Part model, mm, in its own coordinate system. Face numbers are marked on the shaded views. A direction names the side the tool comes from. Round coordinates to 2 decimals unless told otherwise and drop trailing zeros. Loops run counter-clockwise (first coordinate to the right, second up) from the corner with the lowest first, then second, coordinate; pieces in that order, holes last.
(1) Tool access for the marked faces 4, 5 and 6: list every direction of +Z, -Z, +X, -X, +Y, -Y with a clear straight run to the whole face (end or side of a thin tool).
(2) Cut at C-C on x = 13. List the corners of the cut face in (y, z) (3 decimals), then the cut area to 3 significant figures.
(3) Mould opens along X. For the marked faces 1, 2 and 3 say: +X half, -X half, draft (parallel to the pull), parting line (faces both ways), or undercut.
(4) Cut at A-A on z = 7. List the corners of the cut face in (x, y) (3 decimals).
(5) Flat gauge pins, fed straight in: pin 1 (4 mm diameter, centred on x = 10, z = -18, fed in from +Y); pin 2 (0.5 mm diameter, centred on x = -16.5, z = 37, fed in from +Y); pin 3 (1.7 mm diameter, centred on x = -21, z = -35, fed in from +Y). Where does each tip first touch, or does it go through?
(6) Cut at B-B on y = -8. Count the separate pieces of the cut face and the enclosed holes in it, then the cut area to 3 significant figures.
(7) Probe probe 1 along X at (y, z) = (-3.75, 4); probe 2 along Z at (x, y) = (0, -5.5); probe 3 along Z at (x, y) = (-20, -6.25). List the from-to ranges inside material, lowest first.
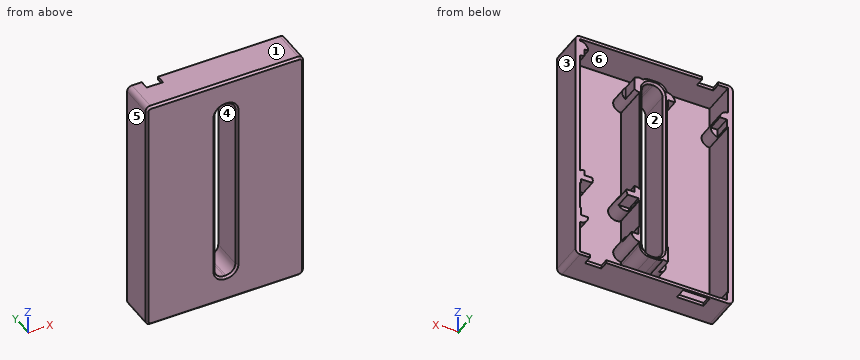
from build123d import *

# Parameters (mm, degrees)
BOSS_EXTRUDE1_DEPTH = 11
SKETCH8_W           = 46
SKETCH8_H           = 73
CUT_EXTRUDE1_DEPTH  = 10.5
BOSS_EXTRUDE2_START = 10.5
SKETCH9_R           = 2.5
BOSS_EXTRUDE2_DEPTH = 10.5
SKETCH10_W          = 15.5
SKETCH10_H          = 43.25
SKETCH10_W_2        = 17.9
SKETCH10_H_2        = 12.3
SKETCH10_W_3        = 18.25
SKETCH10_H_3        = 62
CUT_EXTRUDE3_DEPTH  = 5.25
SKETCH14_W          = 8.25
SKETCH14_H          = 3.5
CUT_EXTRUDE6_DEPTH  = 5
CUT_EXTRUDE7_REACH  = 81.663
SKETCH15_W          = 5.08
SKETCH15_H          = 2.794
CUT_EXTRUDE8_REACH  = 81.663
SKETCH16_W          = 5.08
SKETCH16_H          = 2.794
CHAMFER1_SIZE       = 0.635


with BuildPart() as part:
    # Sketch2 → Boss-Extrude1 (new body)
    with BuildSketch(Plane(origin=(0, 0, 0), x_dir=(1, 0, 0), z_dir=(0, 1, 0))):
        with BuildLine():
            Line((23, -37.5), (-23, -37.5))
            ThreePointArc((-23, -37.5), (-24.060660172, -37.060660172), (-24.5, -36))
            Line((-24.5, -36), (-24.5, 36))
            ThreePointArc((-24.5, 36), (-24.060660172, 37.060660172), (-23, 37.5))
            Line((-23, 37.5), (23, 37.5))
            ThreePointArc((23, 37.5), (24.060660172, 37.060660172), (24.5, 36))
            Line((24.5, 36), (24.5, -36))
            ThreePointArc((24.5, -36), (24.060660172, -37.060660172), (23, -37.5))
        make_face()
        with BuildLine():
            Line((0, 29.5), (0.5, 29.5))
            ThreePointArc((0.5, 29.5), (2.621320344, 28.621320344), (3.5, 26.5))
            Line((3.5, 26.5), (3.5, -26.5))
            ThreePointArc((3.5, -26.5), (2.621320344, -28.621320344), (0.5, -29.5))
            Line((0.5, -29.5), (0, -29.5))
            ThreePointArc((0, -29.5), (-2.121320344, -28.621320344), (-3, -26.5))
            Line((-3, -26.5), (-3, 26.5))
            ThreePointArc((-3, 26.5), (-2.121320344, 28.621320344), (0, 29.5))
        make_face(mode=Mode.SUBTRACT)
    extrude(amount=-BOSS_EXTRUDE1_DEPTH)

    # Sketch8 → Cut-Extrude1 (cut)
    # profile 1 of 2: a face of its own
    with BuildSketch(Plane(origin=(0, 0, 0), x_dir=(1, 0, 0), z_dir=(0, 1, 0))):
        Rectangle(SKETCH8_W, SKETCH8_H)
        with BuildLine():
            Line((-1, 30.5), (1.5, 30.5))
            ThreePointArc((1.5, 30.5), (3.621320344, 29.621320344), (4.5, 27.5))
            Line((4.5, 27.5), (4.5, -27.5))
            ThreePointArc((4.5, -27.5), (3.621320344, -29.621320344), (1.5, -30.5))
            Line((1.5, -30.5), (-1, -30.5))
            ThreePointArc((-1, -30.5), (-3.121320344, -29.621320344), (-4, -27.5))
            Line((-4, -27.5), (-4, 27.5))
            ThreePointArc((-4, 27.5), (-3.121320344, 29.621320344), (-1, 30.5))
        make_face(mode=Mode.SUBTRACT)
    # profile 2 of 2: a face of its own
    with BuildSketch(Plane(origin=(0, 0, 0), x_dir=(1, 0, 0), z_dir=(0, 1, 0))):
        with BuildLine():
            Line((0, 29.5), (0.5, 29.5))
            ThreePointArc((0.5, 29.5), (2.621320344, 28.621320344), (3.5, 26.5))
            Line((3.5, 26.5), (3.5, -26.5))
            ThreePointArc((3.5, -26.5), (2.621320344, -28.621320344), (0.5, -29.5))
            Line((0.5, -29.5), (0, -29.5))
            ThreePointArc((0, -29.5), (-2.121320344, -28.621320344), (-3, -26.5))
            Line((-3, -26.5), (-3, 26.5))
            ThreePointArc((-3, 26.5), (-2.121320344, 28.621320344), (0, 29.5))
        make_face()
    extrude(amount=-CUT_EXTRUDE1_DEPTH, mode=Mode.SUBTRACT)

    # Sketch9 → Boss-Extrude2 (add)
    with BuildSketch(Plane(origin=(0, -10.5, 0), x_dir=(1, 0, 0), z_dir=(0, 1, 0)).offset(BOSS_EXTRUDE2_START)):
        with Locations((21.58, 10.667919779)):
            Circle(SKETCH9_R)
        with Locations((6.08, 10.21529089)):
            Circle(SKETCH9_R)
        with BuildLine():
            Line((24.5, -35.456747529), (24.5, -31.456747529))
            ThreePointArc((24.5, -31.456747529), (20.5, -33.456747529), (24.5, -35.456747529))
        make_face()
        with BuildLine():
            Line((4.5, 26.342587088), (4.5, 21.342587088))
            ThreePointArc((4.5, 21.342587088), (7, 23.842587088), (4.5, 26.342587088))
        make_face()
        with BuildLine():
            Line((-4, 27.5), (-4, 25))
            ThreePointArc((-4, 25), (-6.442500859, 28.033094319), (-2.958333333, 29.772648357))
            ThreePointArc((-2.958333333, 29.772648357), (-3.727178029, 28.75), (-4, 27.5))
        make_face()
        with BuildLine():
            Line((-24.5, -27.605307327), (-24.5, -23.605307327))
            ThreePointArc((-24.5, -23.605307327), (-20.5, -25.605307327), (-24.5, -27.605307327))
        make_face()
        with BuildLine():
            Line((-20.757613835, 37.5), (-23, 37.5))
            ThreePointArc((-23, 37.5), (-24.060660172, 37.060660172), (-24.5, 36))
            Line((-24.5, 36), (-24.5, 34.394692673))
            ThreePointArc((-24.5, 34.394692673), (-21.40359225, 34.470769001), (-20.757613835, 37.5))
        make_face()
        with BuildLine():
            Line((24.5, 21.842587088), (24.5, 25.842587088))
            ThreePointArc((24.5, 25.842587088), (20.5, 23.842587088), (24.5, 21.842587088))
        make_face()
        with BuildLine():
            Line((-4, -23.105307327), (-4, -27.5))
            ThreePointArc((-4, -27.5), (-3.984574172, -27.803837144), (-3.938455326, -28.104549663))
            ThreePointArc((-3.938455326, -28.104549663), (-6.499810577, -25.636081995), (-4, -23.105307327))
        make_face()
        with BuildLine():
            Line((4.5, -25), (4.5, -27.5))
            ThreePointArc((4.5, -27.5), (4.227178029, -28.75), (3.458333333, -29.772648357))
            ThreePointArc((3.458333333, -29.772648357), (6.942500859, -28.033094319), (4.5, -25))
        make_face()
    extrude(amount=-BOSS_EXTRUDE2_DEPTH)

    # Sketch10 → Cut-Extrude3 (cut)
    with BuildSketch(Plane(origin=(0, -5.25, 0), x_dir=(1, 0, 0), z_dir=(0, 1, 0))):
        with Locations((13.83, -11.831747529)):
            Rectangle(SKETCH10_W, SKETCH10_H)
        with Locations((13.825, 17.692587088)):
            Rectangle(SKETCH10_W_2, SKETCH10_H_2)
        with Locations((-13.5, 5.394692673)):
            Rectangle(SKETCH10_W_3, SKETCH10_H_3)
    extrude(amount=CUT_EXTRUDE3_DEPTH, mode=Mode.SUBTRACT)

    # Sketch14 → Cut-Extrude6 (cut)
    with BuildSketch(Plane.XY.offset(-36.5)):
        with Locations((-13.5, -2.4)):
            Rectangle(SKETCH14_W, SKETCH14_H)
    extrude(amount=-CUT_EXTRUDE6_DEPTH, mode=Mode.SUBTRACT)

    # Sketch15 → Cut-Extrude7 (cut, up to next)
    with BuildSketch(Plane(origin=(0, 0, -37.5), x_dir=(-1, 0, 0), z_dir=(0, 0, -1)), mode=Mode.PRIVATE) as cut_extrude7_sk1:
        with Locations((-17.412, -1.397)):
            Rectangle(SKETCH15_W, SKETCH15_H)
    cut_extrude7_tool1 = extrude(cut_extrude7_sk1.sketch, amount=-CUT_EXTRUDE7_REACH, mode=Mode.PRIVATE) & part.part
    add(cut_extrude7_tool1.solids().sort_by_distance((17.412, -1.397, -37.5))[0], mode=Mode.SUBTRACT)

    # Sketch16 → Cut-Extrude8 (cut, up to next)
    with BuildSketch(Plane.XY.offset(37.5), mode=Mode.PRIVATE) as cut_extrude8_sk1:
        with Locations((-17.412, -1.397)):
            Rectangle(SKETCH16_W, SKETCH16_H)
    cut_extrude8_tool1 = extrude(cut_extrude8_sk1.sketch, amount=-CUT_EXTRUDE8_REACH, mode=Mode.PRIVATE) & part.part
    add(cut_extrude8_tool1.solids().sort_by_distance((-17.412, -1.397, 37.5))[0], mode=Mode.SUBTRACT)

    # Chamfer1
    chamfer1_edges = [part.edges().sort_by_distance(p)[0] for p in [
        (-24.060660172, -11, -37.060660172),
        (-24.5, -11, 0),
        (-2.121320344, 0, -28.621320344),
        (-3, 0, 0),
        (-2.121320344, 0, 28.621320344),
        (0.25, 0, 29.5),
        (2.621320344, 0, 28.621320344),
        (3.5, 0, 0),
        (-24.060660172, -11, 37.060660172),
        (2.621320344, 0, -28.621320344),
        (0.25, 0, -29.5),
        (0, -11, 37.5),
        (24.060660172, -11, 37.060660172),
        (24.5, -11, 0),
        (24.060660172, -11, -37.060660172),
        (0.25, -11, -29.5),
        (2.621320344, -11, -28.621320344),
        (3.5, -11, 0),
        (0, -11, -37.5),
        (2.621320344, -11, 28.621320344),
        (0.25, -11, 29.5),
        (-2.121320344, -11, 28.621320344),
        (-3, -11, 0),
        (-2.121320344, -11, -28.621320344),
    ]]
    chamfer(chamfer1_edges, length=CHAMFER1_SIZE)


solid = part.part
Final values:
1. face 4: +Y, -Y
1. face 5: +Z, -Z, -X, +Y, -Y
1. face 6: +Y
2. outline: (-11, -36.865) - (-10.365, -37.5) - (0, -37.5) - (0, -36.5) - (-10.5, -36.5) - (-10.5, 36.5) - (0, 36.5) - (0, 37.5) - (-10.365, 37.5) - (-11, 36.865) - close
2. area: 58.1 mm2
3. face 1: draft
3. face 2: undercut
3. face 3: +X half
4. outline: (-24.5, -10.365) - (-23.865, -11) - (-3.635, -11) - (-3, -10.365) - (-3, -0.635) - (-3.635, 0) - (-4, 0) - (-4, -10.5) - (-23, -10.5) - (-23, 0) - (-24.5, 0) - close; (3.5, -10.365) - (4.135, -11) - (23.865, -11) - (24.5, -10.365) - (24.5, 0) - (23, 0) - (23, -10.5) - (4.5, -10.5) - (4.5, 0) - (4.135, 0) - (3.5, -0.635) - close
5. pin 1: stops at y = -10.5
5. pin 2: stops at y = -2.79
5. pin 3: stops at y = -5.25
6. separate pieces: 2
6. enclosed holes: 2
6. area: 559 mm2
7. probe 1: x = -24.5 to -23, -4 to -3, 3.5 to 4.5, 23 to 24.5
7. probe 2: z = -37.5 to -36.5, -30.5 to -29.5, 29.5 to 30.5, 36.5 to 37.5
7. probe 3: z = -37.5 to -36.5, 36.5 to 37.5
